```python
from build123d import *

# Parameters (mm, degrees)
EXTRUDE_1_DEPTH     = 5
SKETCH_8_OUTSIDE_W  = 22.464
SKETCH_8_OUTSIDE_H  = 20.522
SKETCH_8_OUTSIDE_R  = 6.278684177
CUT_EXTRUDE_1_DEPTH = 1
CUT_EXTRUDE_1_DRAFT = -45
SKETCH_9_R          = 3.825
BOLT_LENGTH_DEPTH   = 30
FILLET_1_R          = 1
CHAMFER_1_SIZE      = 1


with BuildPart() as part:
    # Эскиз6 → Бобышка-Вытянуть1 (new body)
    with BuildSketch(Plane(origin=(0, 0, 0), x_dir=(1, 0, 0), z_dir=(0, 1, 0))):
        Polygon((7.25, 0), (3.625, 6.278684177), (-3.625, 6.278684177), (-7.25, 0), (-3.625, -6.278684177), (3.625, -6.278684177), align=None)
    extrude(amount=EXTRUDE_1_DEPTH)


with BuildPart() as cut_extrude_1_tool:
    # Эскиз8 outside → Вырез-Вытянуть1 (with draft: the straight prism first)
    with BuildSketch(Plane(origin=(0, 5, 0), x_dir=(1, 0, 0), z_dir=(0, 1, 0))):
        Rectangle(SKETCH_8_OUTSIDE_W, SKETCH_8_OUTSIDE_H)
        Circle(SKETCH_8_OUTSIDE_R, mode=Mode.SUBTRACT)
    extrude(amount=-CUT_EXTRUDE_1_DEPTH)
    # Вырез-Вытянуть1: the draft: its side faces are tilted about the plane it starts from
    cut_extrude_1_sides = [cut_extrude_1_tool.faces().sort_by_distance(p)[0] for p in [
        (0, 4.5, 10.261),
        (11.232, 4.5, 0),
        (0, 4.5, -10.261),
        (-11.232, 4.5, 0),
        (-6.278684177, 4.5, 0),
    ]]
    draft(cut_extrude_1_sides, Plane(origin=(0, 5, 0), x_dir=(1, 0, 0), z_dir=(0, 1, 0)), CUT_EXTRUDE_1_DRAFT)


with BuildPart() as part_1:
    add(part.part)

    # Вырез-Вытянуть1: cut by cut_extrude_1_tool
    add(cut_extrude_1_tool.part, mode=Mode.SUBTRACT)

    # Эскиз9 → bolt length (add)
    with BuildSketch(Plane.XZ):
        with Locations(Location((0, 0, 0), (0, 0, 90))):  # turned: the seam where the file's is
            Circle(SKETCH_9_R)
    extrude(amount=BOLT_LENGTH_DEPTH)

    # Скругление1
    fillet_1_edges = [part_1.edges().sort_by_distance(p)[0] for p in [
        (0, 0, -3.825),
    ]]
    fillet(fillet_1_edges, radius=FILLET_1_R)

    # Фаска1
    chamfer_1_edges = [part_1.edges().sort_by_distance(p)[0] for p in [
        (0, -30, -3.825),
    ]]
    chamfer(chamfer_1_edges, length=CHAMFER_1_SIZE)


solid = part_1.part
```
Design review of the part built by this model. Coordinates are the model's own, in mm. A direction names the side the tool comes from. Round coordinates to 2 decimals unless told otherwise and drop trailing zeros. Write each loop counter-clockwise with the first axis right and the second up, starting at its lowest first coordinate (ties: lowest second). Pieces come first, ordered by that corner, then holes. Notation, with made-up numbers: (-27, 85.5) -> (-18, 85.5) arc R38 ccw to (-18, 123.5) -> close; hole circle Ø1 at (-11.5, -13). An arc over 180 degrees is marked (long way). Answer in a Markdown table with one row per item.
Q1. Take a section at A-A, the plane y = -18.5. State the section outline as (x, z) points (3 decimals), then the cut area to 3 significant figures.
The answers:
| item | result |
|---|---|
| outline | circle Ø7.65 at (0, 0) |
| area | 46.0 mm² |
Q2. For faces 1 (the face through (3.241, 4.768, 5.646)), 2 (the face through (3, 0, 4)), list the 3-axis set-ups (+Z, -Z, +X, -X, +Y, -Y) from which the entire face can be reached by the end or side of a thin tool; tool diameter is ignored.
The answers:
| item | result |
|---|---|
| face 1 | +Z, +X, +Y |
| face 2 | -Y |
Q3. Clearance check with flat-ended pins moving along their axes: pin 1 Ø8 at (x, y) = (1, -4.5) entering from +Z; pin 2 Ø6 at (y, z) = (-13, 2) entering from -X (3 decimals); pin 3 Ø1.5 at (y, z) = (1, 1) entering from +X. State where each tip first meets the part, or that it passes through.
The answers:
| item | result |
|---|---|
| pin 1 | z = 3.91 |
| pin 2 | x = -3.825 |
| pin 3 | x = 7.11 |
Q4. To check wall thickness, follow L1, parallel to X at y = -14.5, z = -0.25; L2, parallel to Y at x = 2, z = 4.25; L3, parallel to Z at x = 2.25, y = -19. State the ranges of each line that lie inside material, in increasing order. Write a range as [from, to].
The answers:
| item | result |
|---|---|
| L1 | [-3.82, 3.82] |
| L2 | [-0.01, 5] |
| L3 | [-3.09, 3.09] |
